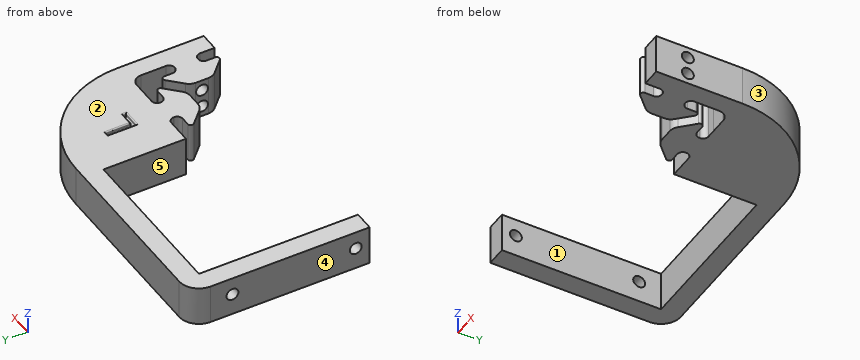
from build123d import *

# Parameters (mm, degrees)
BOSS_EXTRUDE1_DEPTH = 10
CUT_EXTRUDE1_REACH  = 86.489
SKETCH2_R           = 1.5
FILLET3_R           = 5
CUT_EXTRUDE2_REACH  = 86.489
SKETCH3_R           = 1.5
FILLET4_R           = 25
CUT_EXTRUDE7_DEPTH  = 1
FILLET8_R           = 0.3


with BuildPart() as part:
    # Sketch1 → Boss-Extrude1 (new body)
    with BuildSketch(Plane.XY):
        with BuildLine():
            Line((13.02, -7.9417418), (17.7, -7.9417418))
            Line((17.7, -7.9417418), (17.7, 38.77))
            Line((17.7, 38.77), (-56.7, 38.77))
            Line((-56.7, 38.77), (-56.7, -6.23))
            Line((-56.7, -6.23), (-51.7, -6.23))
            Line((-51.7, -6.23), (-51.7, 33.77))
            Line((-51.7, 33.77), (-10.566443095, 33.77))
            Line((-10.566443095, 33.77), (-10.566443095, 13.02))
            Line((-10.566443095, 13.02), (-5.317126718, 13.02))
            Line((-5.317126718, 13.02), (-4.287512407, 13.02))
            ThreePointArc((-4.287512407, 13.02), (-3.319474451, 12.619025549), (-2.9185, 11.650987593))
            Line((-2.9185, 11.650987593), (-2.9185, 11.539212407))
            ThreePointArc((-2.9185, 11.539212407), (-3.319474451, 10.571174451), (-4.287512407, 10.1702))
            Line((-4.287512407, 10.1702), (-6.476788598, 10.1702))
            ThreePointArc((-6.476788598, 10.1702), (-7.136510935, 9.729114651), (-6.981020848, 8.950903446))
            Line((-6.981020848, 8.950903446), (-3.672257405, 5.649701928))
            ThreePointArc((-3.672257405, 5.649701928), (-2.746830644, 5.032499411), (-1.655778399, 4.8158))
            Line((-1.655778399, 4.8158), (1.655778399, 4.8158))
            ThreePointArc((1.655778399, 4.8158), (2.746830644, 5.032499411), (3.672257405, 5.649701928))
            Line((3.672257405, 5.649701928), (6.981020848, 8.950903446))
            ThreePointArc((6.981020848, 8.950903446), (7.136510935, 9.729114651), (6.476788598, 10.1702))
            Line((6.476788598, 10.1702), (4.287512407, 10.1702))
            ThreePointArc((4.287512407, 10.1702), (3.319474451, 10.571174451), (2.9185, 11.539212407))
            Line((2.9185, 11.539212407), (2.9185, 11.650987593))
            ThreePointArc((2.9185, 11.650987593), (3.319474451, 12.619025549), (4.287512407, 13.02))
            Line((4.287512407, 13.02), (6.332886163, 13.02))
            Line((6.332886163, 13.02), (10.562594215, 13.019824354))
            ThreePointArc((10.562594215, 13.019824354), (12.303594776, 12.313982883), (13.019956614, 10.577284622))
            Line((13.019956614, 10.577284622), (13.02, 4.287469289))
            ThreePointArc((13.02, 4.287469289), (12.619025549, 3.319431332), (11.650987593, 2.918456882))
            Line((11.650987593, 2.918456882), (11.539212407, 2.918456882))
            ThreePointArc((11.539212407, 2.918456882), (10.571174451, 3.319431332), (10.1702, 4.287469289))
            Line((10.1702, 4.287469289), (10.1702, 6.402089023))
            ThreePointArc((10.1702, 6.402089023), (9.733877283, 7.055496588), (8.963146507, 6.90287605))
            Line((8.963146507, 6.90287605), (5.667020993, 3.614283579))
            ThreePointArc((5.667020993, 3.614283579), (5.046449321, 2.687255303), (4.8285, 1.593185507))
            Line((4.8285, 1.593185507), (4.8285, -1.593185507))
            ThreePointArc((4.8285, -1.593185507), (5.046449321, -2.687255303), (5.667020993, -3.614283579))
            Line((5.667020993, -3.614283579), (8.963146507, -6.90287605))
            ThreePointArc((8.963146507, -6.90287605), (9.733877283, -7.055496588), (10.1702, -6.402089023))
            Line((10.1702, -6.402089023), (10.1702, -4.287469289))
            ThreePointArc((10.1702, -4.287469289), (10.571174451, -3.319431332), (11.539212407, -2.918456882))
            Line((11.539212407, -2.918456882), (11.650987593, -2.918456882))
            ThreePointArc((11.650987593, -2.918456882), (12.619025549, -3.319431332), (13.02, -4.287469289))
            Line((13.02, -4.287469289), (13.02, -5.3170836))
            Line((13.02, -5.3170836), (13.02, -7.9417418))
        make_face()
    extrude(amount=BOSS_EXTRUDE1_DEPTH)

    # Sketch2 → Cut-Extrude1 (cut, up to next)
    with BuildSketch(Plane.ZY.offset(56.7), mode=Mode.PRIVATE) as cut_extrude1_sk1:
        with Locations((5.5, -2.73)):
            Circle(SKETCH2_R)
    cut_extrude1_tool1 = extrude(cut_extrude1_sk1.sketch, amount=-CUT_EXTRUDE1_REACH, mode=Mode.PRIVATE) & part.part
    # Sketch2 → Cut-Extrude1 (cut, up to next)
    with BuildSketch(Plane.ZY.offset(56.7), mode=Mode.PRIVATE) as cut_extrude1_sk2:
        with Locations((5.5, 28.27)):
            Circle(SKETCH2_R)
    cut_extrude1_tool2 = extrude(cut_extrude1_sk2.sketch, amount=-CUT_EXTRUDE1_REACH, mode=Mode.PRIVATE) & part.part
    add(cut_extrude1_tool1.solids().sort_by_distance((-56.7, -2.73, 5.5))[0], mode=Mode.SUBTRACT)
    add(cut_extrude1_tool2.solids().sort_by_distance((-56.7, 28.27, 5.5))[0], mode=Mode.SUBTRACT)

    # Fillet3
    fillet3_edges = [part.edges().sort_by_distance(p)[0] for p in [
        (-56.7, 38.77, 5),
    ]]
    fillet(fillet3_edges, radius=FILLET3_R)

    # Sketch3 → Cut-Extrude2 (cut, up to next)
    with BuildSketch(Plane(origin=(17.7, 0, 0), x_dir=(0, 0, -1), z_dir=(1, 0, 0)), mode=Mode.PRIVATE) as cut_extrude2_sk1:
        with Locations((-7.25, 0)):
            Circle(SKETCH3_R)
    cut_extrude2_tool1 = extrude(cut_extrude2_sk1.sketch, amount=-CUT_EXTRUDE2_REACH, mode=Mode.PRIVATE) & part.part
    # Sketch3 → Cut-Extrude2 (cut, up to next)
    with BuildSketch(Plane(origin=(17.7, 0, 0), x_dir=(0, 0, -1), z_dir=(1, 0, 0)), mode=Mode.PRIVATE) as cut_extrude2_sk2:
        with Locations(Location((-2.75, 0, 0), (0, 0, 90))):
            Circle(SKETCH3_R)
    cut_extrude2_tool2 = extrude(cut_extrude2_sk2.sketch, amount=-CUT_EXTRUDE2_REACH, mode=Mode.PRIVATE) & part.part
    add(cut_extrude2_tool1.solids().sort_by_distance((17.7, 0, 7.25))[0], mode=Mode.SUBTRACT)
    add(cut_extrude2_tool2.solids().sort_by_distance((17.7, 0, 2.75))[0], mode=Mode.SUBTRACT)

    # Fillet4
    fillet4_edges = [part.edges().sort_by_distance(p)[0] for p in [
        (17.7, 38.77, 5),
    ]]
    fillet(fillet4_edges, radius=FILLET4_R)

    # Sketch7 → Cut-Extrude7 (cut)
    with BuildSketch(Plane.XY.offset(10)):
        Polygon((-0.90100078, 19.84300121), (-0.90100078, 27.034293528), (0.113155829, 27.034293528), (0.113155829, 20.672765708), (3.524409877, 20.672765708), (3.524409877, 19.84300121), align=None)
    extrude(amount=-CUT_EXTRUDE7_DEPTH, mode=Mode.SUBTRACT)

    # Fillet8
    fillet8_edges = [part.edges().sort_by_distance(p)[0] for p in [
        (1.311704549, 19.84300121, 10),
        (-0.90100078, 23.438647369, 10),
        (-0.393922475, 27.034293528, 10),
        (0.113155829, 23.853529618, 10),
        (1.818782853, 20.672765708, 10),
        (3.524409877, 20.257883459, 10),
        (1.311704549, 19.84300121, 9),
        (-0.90100078, 23.438647369, 9),
        (-0.393922475, 27.034293528, 9),
        (0.113155829, 23.853529618, 9),
        (1.818782853, 20.672765708, 9),
        (3.524409877, 20.257883459, 9),
    ]]
    fillet(fillet8_edges, radius=FILLET8_R)


solid = part.part
The model under review builds one solid part; all positions refer to its coordinate system, in mm. Face numbers are marked on the shaded views. A direction names the side the tool comes from. Round coordinates to 2 decimals unless told otherwise and drop trailing zeros. Order: outer loops, then holes, each group sorted by start corner. A loop starts at its lowest first (then second) coordinate and runs counter-clockwise, first axis right, second up. Notation, with made-up numbers: (89, 72) -> (129, 72) arc R26 cw to (129, 95) -> close; hole circle Ø10 at (62, -11.5). An arc over 180 degrees is marked (long way). Return JSON: item names as keys, results as strings.
1. The part is to be moulded in two halves that separate along X. For the marked faces 1, 2 and 3, say which applies: +X half, -X half, draft (parallel to the pull), parting line (faces both ways), or undercut.
Answer block:
{"face 1": "undercut", "face 2": "draft", "face 3": "+X half"}
2. Take a section at D-D (z = 5). State how many separate pieces and enclosed holes the cut face has, then the cut area to 3 significant figures.
Answer block:
{"separate pieces": "3", "enclosed holes": "0", "area": "1,240 mm²"}
3. Insertion check: P1, Ø4, axis at x = -54.5, z = 7, coming from the -Y side; P2, Ø1.5, axis at x = -34, z = 2, coming from the -Y side; P3, Ø3.5, axis at x = 8, z = 6.5, coming from the -Y side; P4, Ø1, axis at x = -42, y = 32.5, coming from the -Z side. Each pin has a flat end and moves straight along its axis. Give the tip position at first contact, or say it passes through.
Answer block:
{"P1": "stops at y = -6.23", "P2": "stops at y = 33.77", "P3": "stops at y = -7.11", "P4": "passes through"}
4. Take a section at B-B (y = 28.27). Write out the cut boundary in (x, z).
Answer block:
{"outline": "(-56.7, 0) -> (-51.7, 0) -> (-51.7, 4) -> (-56.7, 4) -> close; (-56.7, 7) -> (-51.7, 7) -> (-51.7, 10) -> (-56.7, 10) -> close; (-10.57, 0) -> (13.07, 0) -> (13.07, 10) -> (-10.57, 10) -> close"}
5. Take a section at C-C (x = -31.5). Write out the cut boundary in (y, z).
Answer block:
{"outline": "(33.77, 0) -> (38.77, 0) -> (38.77, 10) -> (33.77, 10) -> close"}
6. For the marked faces 4 and 5, list the 3-axis set-ups (+Z, -Z, +X, -X, +Y, -Y) from which the entire face can be reached by the end or side of a thin tool; tool diameter is ignored.
Answer block:
{"face 4": "+Z, -Z, -X, +Y, -Y", "face 5": "+Z, -Z, -Y"}
7. Take a section at A-A (y = 0). Write out the cut boundary in (x, z).
Answer block:
{"outline": "(-56.7, 0) -> (-51.7, 0) -> (-51.7, 10) -> (-56.7, 10) -> close; (4.83, 0) -> (17.7, 0) -> (17.7, 1.25) -> (4.83, 1.25) -> close; (4.83, 4.25) -> (17.7, 4.25) -> (17.7, 5.75) -> (4.83, 5.75) -> close; (4.83, 8.75) -> (17.7, 8.75) -> (17.7, 10) -> (4.83, 10) -> close"}
8. For L1, parallel to Y at x = -54.65, z = 5.5; L2, parallel to X at y = 8.5, z = 7; L3, parallel to X at y = 3.5, z = 9.5, list the stretches that pass through material, from the lowest coordinate up. Write a range as [from, to].
Answer block:
{"L1": "y = [-6.23, -4.23], [-1.23, 26.77], [29.77, 37.81]", "L2": "x = [-56.7, -51.7], [-6.53, 6.53], [13.02, 17.7]", "L3": "x = [-56.7, -51.7], [5.56, 10.42], [12.77, 17.7]"}
